Part model, mm, in its own coordinate system. Round coordinates to 2 decimals unless told otherwise and drop trailing zeros. Write each loop counter-clockwise with the first axis right and the second up, starting at its lowest first coordinate (ties: lowest second). Pieces come first, ordered by that corner, then holes. Notation, with made-up numbers: (57.25, 28.5) -> (64.25, 28.5) arc R18 ccw to (64.25, 62.5) -> close; hole circle Ø11 at (43, 8.25). An arc over 180 degrees is marked (long way). Return JSON: item names as keys, results as strings. Group by question number.
(1) Saw through at A-A (z = 5). List the corners of the cut face in (x, y).
(2) Saw through at D-D (y = 58). List the corners of the cut face in (x, z), plus the area to 3 significant figures.
(3) Saw through at B-B (y = 85.5). List the corners of the cut face in (x, z), plus the area to 3 significant figures.
(4) Drop flat-ended pins along their axis: pin 1 Ø6 at (y, z) = (43, 9) entering from +X; pin 2 Ø3 at (y, z) = (97, 4) entering from -X; pin 3 Ø1 at (x, y) = (12.5, 72) entering from -Z; pin 4 Ø5 at (x, z) = (27, 3) entering from -Y. Give the stop position or say it passes through.
(5) Drill centre lines: L1, parallel to Y at x = 27.5, z = 6; L2, parallel to Y at x = -21, z = 8.75; L3, parallel to X at y = -22.5, z = 3.5. Where is each one in solid material? Low to high. Write a range as from..to.
(6) Saw through at C-C (x = 10). List the corners of the cut face in (y, z), plus the area to 3 significant figures.
from build123d import *

# Parameters (mm, degrees)
BOSS_EXTRUDE1_DEPTH      = 10
BOSS_EXTRUDE1_DEPTH_BACK = 0.318278283
SKETCH3_R                = 3
CUT_EXTRUDE1_DEPTH       = 5
CUT_EXTRUDE2_DEPTH       = 15


with BuildPart() as part:
    # Sketch2 → Boss-Extrude1 (new body, two sides)
    with BuildSketch(Plane.XY) as boss_extrude1_sk:
        Polygon((14.539831303, 82.09905821), (-41.416945568, -37.900637039), (-51.156779582, -33.358877849), (7.345216778, 92.09905821), (7.345216778, 102.09905821), (47.345216778, 102.09905821), (47.345216778, 82.09905821), align=None)
    extrude(amount=BOSS_EXTRUDE1_DEPTH)
    extrude(boss_extrude1_sk.sketch, amount=-BOSS_EXTRUDE1_DEPTH_BACK)

    # Sketch3 → Cut-Extrude1 (cut)
    with BuildSketch(Plane.XZ.offset(-82.09905821)):
        with Locations((37.223217292, 5)):
            Circle(SKETCH3_R)
    extrude(amount=-CUT_EXTRUDE1_DEPTH, mode=Mode.SUBTRACT)

    # Sketch4 → Cut-Extrude2 (cut)
    with BuildSketch(Plane(origin=(0, 0, -0.318278283), x_dir=(-1, 0, 0), z_dir=(0, 0, -1))):
        Polygon((51.156779582, -33.358877849), (39.299088476, -33.358877849), (41.416945568, -37.900637039), align=None)
    extrude(amount=-CUT_EXTRUDE2_DEPTH, mode=Mode.SUBTRACT)


solid = part.part
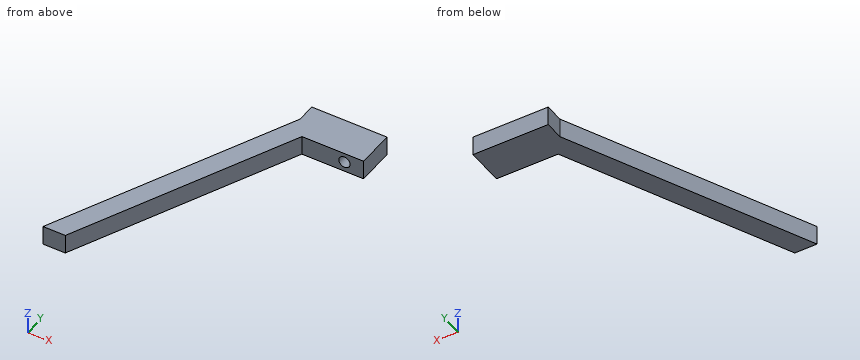
Computed values:
{
 "1": {"outline": "(-51.16, -33.36) -> (-39.3, -33.36) -> (14.54, 82.1) -> (34.22, 82.1) -> (34.22, 87.1) -> (40.22, 87.1) -> (40.22, 82.1) -> (47.35, 82.1) -> (47.35, 102.1) -> (7.35, 102.1) -> (7.35, 92.1) -> close"},
 "2": {"outline": "(-8.56, -0.32) -> (3.3, -0.32) -> (3.3, 10) -> (-8.56, 10) -> close", "area": "122 mm2"},
 "3": {"outline": "(4.27, -0.32) -> (47.35, -0.32) -> (47.35, 10) -> (4.27, 10) -> close; hole circle Ø6 at (37.22, 5)", "area": "416 mm2"},
 "4": {"pin 1": "x = -2.29", "pin 2": "x = 7.35", "pin 3": "through", "pin 4": "y = 82.1"},
 "5": {"L1": "82.1..102.1", "L2": "5.88..31.31", "L3": "-46.09..-34.24"},
 "6": {"outline": "(72.36, -0.32) -> (102.1, -0.32) -> (102.1, 10) -> (72.36, 10) -> close", "area": "307 mm2"}
}
